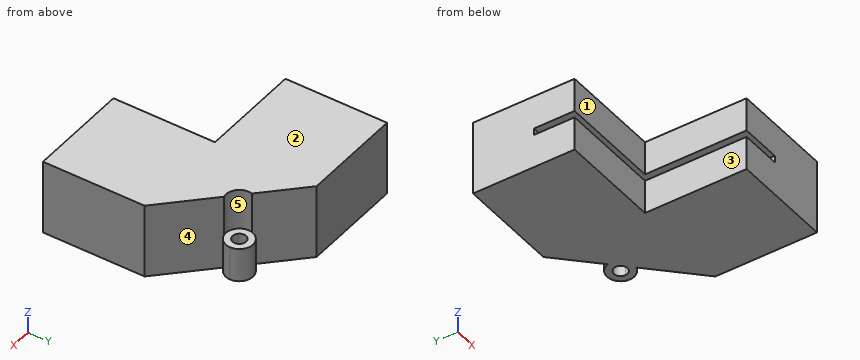
```python
from build123d import *

# Parameters (mm, degrees)
F0_W     = 30
F0_H     = 30
F1_DEPTH = 12
F2_W     = 12
F2_H     = 30
F2_H_2   = 12
F2_W_2   = 30
F3_DEPTH = 3.5
F4_W     = 30
F4_H     = 12
F4_W_2   = 12
F4_H_2   = 30
F4_H_3   = 18
F4_W_3   = 18
F5_DEPTH = 10
F6_DEPTH = 10


with BuildPart() as f1:
    # F0 (on Top) → F1 (new body)
    with BuildSketch(Plane.XY):
        with Locations((15, -15)):
            Rectangle(F0_W, F0_H)
        with BuildLine():
            Line((0, 30), (0, 0))
            Line((0, 0), (30, 0))
            Line((30, 0), (16.1747587326, 13.8252412674))
            ThreePointArc((16.1747587326, 13.8252412674), (12.3110554274, 14.8605174478), (11.275779247, 18.724220753))
            Line((11.275779247, 18.724220753), (0, 30))
        make_face()
        with Locations((-15, 15)):
            Rectangle(F0_W, F0_H)
    extrude(amount=F1_DEPTH)

    # F2 (on face) → F3 (cut)
    with BuildSketch(Plane.XY.offset(12)):
        with Locations((6, -15)):
            Rectangle(F2_W, F2_H)
        with Locations((6, 6)):
            Rectangle(F2_W, F2_H_2)
        with Locations((-15, 6)):
            Rectangle(F2_W_2, F2_H_2)
    extrude(amount=-F3_DEPTH, mode=Mode.SUBTRACT)

    # F4 (on face) → F5 (join)
    with BuildSketch(Plane.XY.offset(12)):
        with Locations((-15, 6)):
            Rectangle(F4_W, F4_H)
        with Locations((6, -15)):
            Rectangle(F4_W_2, F4_H_2)
        with BuildLine():
            Line((11.275779247, 18.724220753), (0, 30))
            Line((0, 30), (0, 12))
            Line((0, 12), (12, 12))
            Line((12, 12), (12, 0))
            Line((12, 0), (30, 0))
            Line((30, 0), (16.1747587326, 13.8252412674))
            ThreePointArc((16.1747587326, 13.8252412674), (12.3110554274, 14.8605174478), (11.275779247, 18.724220753))
        make_face()
        with Locations((6, 6)):
            Rectangle(F4_W_2, F4_H)
        with Locations((-15, 21)):
            Rectangle(F4_W, F4_H_3)
        with Locations((21, -15)):
            Rectangle(F4_W_3, F4_H_2)
    extrude(amount=F5_DEPTH)

    # F0 (on Top) → F6 (join)
    with BuildSketch(Plane.XY):
        with Locations((-15, 15)):
            Rectangle(F0_W, F0_H)
        with BuildLine():
            Line((0, 30), (0, 0))
            Line((0, 0), (30, 0))
            Line((30, 0), (16.1747587326, 13.8252412674))
            ThreePointArc((16.1747587326, 13.8252412674), (12.3110554274, 14.8605174478), (11.275779247, 18.724220753))
            Line((11.275779247, 18.724220753), (0, 30))
        make_face()
        with Locations((15, -15)):
            Rectangle(F0_W, F0_H)
        with BuildLine():
            ThreePointArc((19.1394825522, 17.6889445726), (15.6615873211, 21.6547240181), (11.275779247, 18.724220753))
            Line((11.275779247, 18.724220753), (13.7252689898, 16.2747310102))
            Line((13.7252689898, 16.2747310102), (16.1747587326, 13.8252412674))
            ThreePointArc((16.1747587326, 13.8252412674), (18.3128959133, 15.2538988565), (19.1394825522, 17.6889445726))
        make_face()
        with BuildLine():
            ThreePointArc((17.1394825522, 17.6889445726), (15.9048494169, 15.8411855075), (13.7252689898, 16.2747310102))
            ThreePointArc((13.7252689898, 16.2747310102), (14.3741156874, 19.5367036376), (17.1394825522, 17.6889445726))
        make_face(mode=Mode.SUBTRACT)
        with BuildLine():
            Line((13.7252689898, 16.2747310102), (11.275779247, 18.724220753))
            ThreePointArc((11.275779247, 18.724220753), (12.3110554274, 14.8605174478), (16.1747587326, 13.8252412674))
            Line((16.1747587326, 13.8252412674), (13.7252689898, 16.2747310102))
        make_face()
    extrude(amount=F6_DEPTH)


solid = f1.part
```
Design review of the part built by this model. Coordinates are the model's own, in mm. Face numbers are marked on the shaded views. A direction names the side the tool comes from. Round coordinates to 2 decimals unless told otherwise and drop trailing zeros. Order: outer loops, then holes, each group sorted by start corner. A loop starts at its lowest first (then second) coordinate and runs counter-clockwise, first axis right, second up. Notation, with made-up numbers: M -19.75,45.25 L -12.75,45.25 A20 ccw -12.75,71.25 Z; hole C 36.25,27 d10. An arc over 180 degrees is marked long. Put each result on its own line as item: value.
Q1. Consider section B-B (y = 4). State the section outline as (x, z) points, and give its area (3 significant figures).
Reported:
outline: M -30,0 L 26,0 L 26,22 L -30,22 L -30,12 L 12,12 L 12,10 L -30,10 Z
area: 1,150 mm²
Q2. Consider section C-C (x = -2.5). State the section outline as (y, z) points, and give its area (3 significant figures).
Reported:
outline: M 0,0 L 30,0 L 30,22 L 0,22 L 0,12 L 12,12 L 12,10 L 0,10 Z
area: 636 mm²
Q3. Draft analysis for pull direction X (two halves, no side actions). For the marked faces 3, 4 and 5, state which applies: released by +X, released by -X, zero draft, split by the parting line, or undercut.
Reported:
face 3: released by -X
face 4: released by +X
face 5: undercut
Q4. Consider section A-A (z = 16.75). State the section outline as (x, y) points, and give its area (3 significant figures).
Reported:
outline: M -30,0 L 0,0 L 0,-30 L 30,-30 L 30,0 L 16.17,13.83 A4 cw 11.28,18.72 L 0,30 L -30,30 Z
area: 2,240 mm²
Q5. Insertion check: pin 1 Ø4 at (y, z) = (-14.5, 13) entering from -X; pin 2 Ø5 at (y, z) = (5.5, 2.5) entering from +X; pin 3 Ø10 at (x, z) = (-11, 2.5) entering from -Y. Each pin has a flat end and moves straight along its axis. Give the tip position at first contact, or say it passes through.
Reported:
pin 1: x = 0
pin 2: x = 27
pin 3: y = 0
Q6. Consider section D-D (z = 4.25). State the section outline as (x, y) points, and give its area (3 significant figures).
Reported:
outline: M -30,0 L 0,0 L 0,-30 L 30,-30 L 30,0 L 16.17,13.83 A4 ccw long 11.28,18.72 L 0,30 L -30,30 Z; hole C 15.14,17.69 d4
area: 2,280 mm²
Q7. To check wall thickness, follow line 1 (X direction, y = 20, z = 11.5); line 2 (X direction, y = -25, z = 12.25); line 3 (Z direction, x = 1, y = -13). State the ranges of each line that lie inside material, in increasing order.
Reported:
line 1: -30 to 10
line 2: 0 to 30
line 3: 0 to 10, 12 to 22
Q8. Machinability: for the marked faces 1 and 2, which of the approach directions +Z, -Z, +X, -X, +Y, -Y give a long, thin tool a straight path to every point of the face, cutting with its end or side? Answer none if there is none.
Reported:
face 1: +Z, -Z, -X, -Y
face 2: +Z, +X, -X, +Y, -Y
